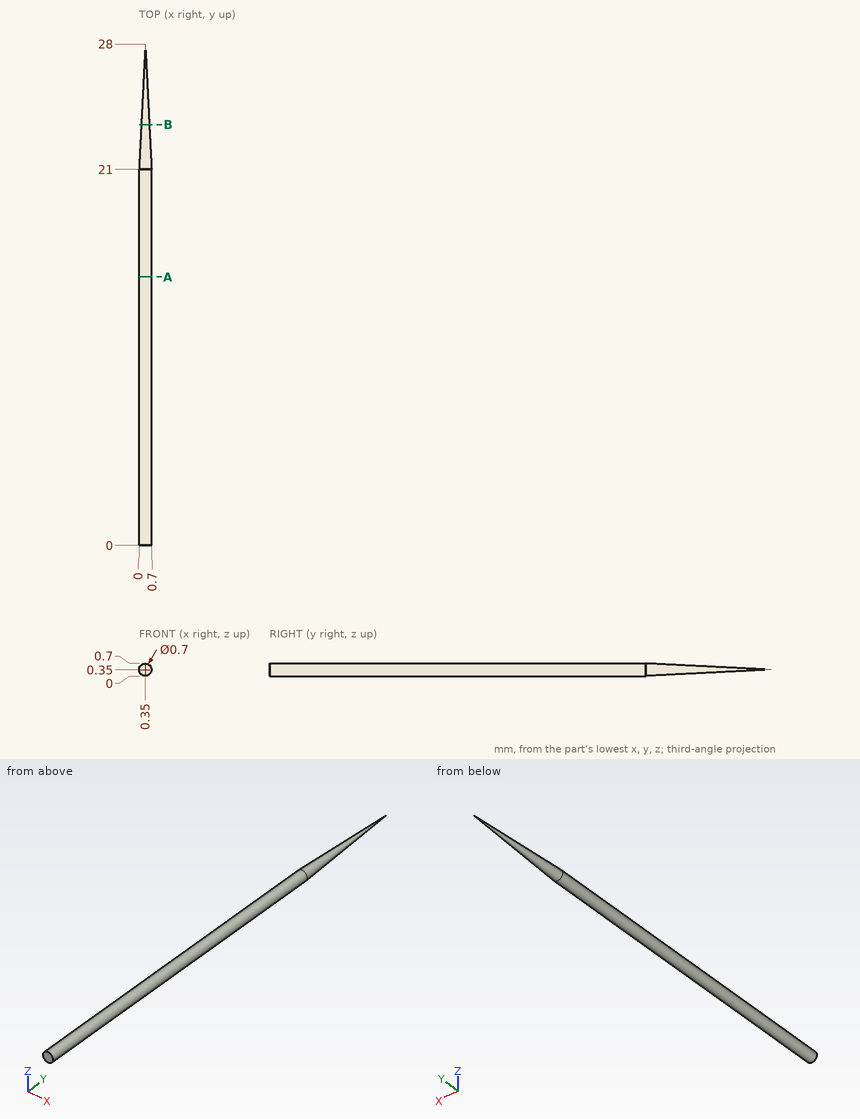
Design review of the part shown in the three views and the two pictorial views. Dimensions are in mm from the part's minimum x, y and z. Give positions to 0.01 mm unless a question says otherwise; leave off trailing zeros. Loops run counter-clockwise (first coordinate to the right, second up) from the corner with the lowest first, then second, coordinate; pieces in that order, holes last. Notation, with made-up numbers: M 23.25,88 L 29.25,88 A17 cw 29.25,108 Z; hole C -22,-20.5 d8. An arc over 180 degrees is marked long. Write item = value, one per line.
Q1. We need section A-A (y = 15). Give the boundary of the cut face in (x, z), plus the area to 3 significant figures.
Output values:
outline = C 0.35,0.35 d0.7
area = 0.385 mm^2
Q2. To check wall thickness, follow line 1 (X direction, y = 17, z = 0.4); line 2 (Z direction, x = 0.1, y = 2). State the ranges of each line that lie inside material, in increasing order. Write a range as [from, to].
Output values:
line_1 = [0, 0.7]
line_2 = [0.11, 0.59]
Q3. We need section B-B (y = 23.5). Give the boundary of the cut face in (x, z) (3 decimals), plus the area to 3 significant figures.
Output values:
outline = C 0.35,0.35 d0.45
area = 0.159 mm^2
